Here's how the part is built. I have some questions about the finished solid (model axes, mm). A direction names the side the tool comes from. Give positions to 0.01 mm unless a question says otherwise; leave off trailing zeros. Write each loop counter-clockwise with the first axis right and the second up, starting at its lowest first coordinate (ties: lowest second). Pieces come first, ordered by that corner, then holes. Notation, with made-up numbers: (-22.75, 7.25) - (-18.75, 7.25) arc R12 cw to (-18.75, 22.25) - close; hole circle Ø9 at (14, 13.25). An arc over 180 degrees is marked (long way). Use a Markdown table: item, result.
```python
from build123d import *

# Parameters (mm, degrees)
SKETCH1_R           = 9
SKETCH1_R_2         = 3
BOSS_EXTRUDE1_DEPTH = 40
SKETCH2_W           = 5
SKETCH2_H           = 5


with BuildPart() as part:
    # Sketch1 → Boss-Extrude1 (new body)
    with BuildSketch(Plane(origin=(0, 0, 0), x_dir=(0, 0, -1), z_dir=(1, 0, 0))):
        Circle(SKETCH1_R)
        Circle(SKETCH1_R_2, mode=Mode.SUBTRACT)
    extrude(amount=BOSS_EXTRUDE1_DEPTH)

    # Sketch2 → Cut-Revolve1 (revolve, cut)
    with BuildSketch(Plane.XY, mode=Mode.PRIVATE) as cut_revolve1_sk:
        with Locations((2.5, 6.5)):
            Rectangle(SKETCH2_W, SKETCH2_H)
        with Locations((37.5, 6.5)):
            Rectangle(SKETCH2_W, SKETCH2_H)
    revolve(cut_revolve1_sk.sketch.rotate(Axis((0, 0, 0), (1, 0, 0)), 90), axis=Axis((0, 0, 0), (1, 0, 0)), mode=Mode.SUBTRACT)


solid = part.part
```
Item 1: Thinking about a two-plate mould opening in Y: for faces 1 (the cylindrical face through (2.535, 3.905, -0.867)), 2 (the flat face through (35, 4, -2)), 3 (the cylindrical face through (20, 0, 3)), which applies, +Y half, -Y half, draft (parallel to the pull), parting line (faces both ways), or undercut?
Values:
| item | result |
|---|---|
| face 1 | parting line |
| face 2 | draft |
| face 3 | undercut |
Item 2: Will these pins go through, and if not, where does the flat tip stop? pin 1 Ø9 at (y, z) = (3, 3) entering from -X; pin 2 Ø1 at (x, z) = (27.5, -2.5) entering from +Y; pin 3 Ø5 at (x, z) = (35.5, -5) entering from +Y; pin 4 Ø5 at (x, y) = (24, -4) entering from +Z.
Values:
| item | result |
|---|---|
| pin 1 | stops at x = 0 |
| pin 2 | stops at y = 8.77 |
| pin 3 | stops at y = 8.63 |
| pin 4 | stops at z = 8.87 |
Item 3: I need wall thicknesses on line 1 along Y through (x, z) = (13.5, 0); line 2 along X through (y, z) = (5.75, -2.5); line 3 along Y through (x, z) = (10, -2.5). Which ranges of each line are inside material? Lowest first, please. Write a range as [from, to].
Values:
| item | result |
|---|---|
| line 1 | y = [-9, -3], [3, 9] |
| line 2 | x = [5, 35] |
| line 3 | y = [-8.65, -1.66], [1.66, 8.65] |
Item 4: If we section it at C-C, the plane x = 12: Write out the boundary of the cut face in (y, z).
Values:
| item | result |
|---|---|
| outline | circle Ø18 at (0, 0); hole circle Ø6 at (0, 0) |
Item 5: If we section it at D-D, the plane z = -5: Write out the boundary of the cut face in (x, y), plus the area to 3 significant figures.
Values:
| item | result |
|---|---|
| outline | (5, -7.48) - (35, -7.48) - (35, 7.48) - (5, 7.48) - close |
| area | 449 mm2 |
Item 6: For faces 4 (the cylindrical face through (37.535, 3.905, -0.867)), 5 (the flat face through (40, 3, -1)), 6 (the flat face through (5, 4, -2)), which set-ups out of +Z, -Z, +X, -X, +Y, -Y let a thin tool reach every point of the face, with its end or its side?
Values:
| item | result |
|---|---|
| face 4 | +X |
| face 5 | +Z, -Z, +X, +Y, -Y |
| face 6 | -X |
Item 7: If we section it at A-A, the plane y = 0: Write out the boundary of the cut face in (x, z).
Values:
| item | result |
|---|---|
| outline | (0, -4) - (5, -4) - (5, -9) - (35, -9) - (35, -4) - (40, -4) - (40, -3) - (0, -3) - close; (0, 3) - (40, 3) - (40, 4) - (35, 4) - (35, 9) - (5, 9) - (5, 4) - (0, 4) - close |
